```python
from build123d import *

# Parameters (mm, degrees)
CROQUIS1_W              = 66
CROQUIS1_H              = 62
SALIENTE_EXTRUIR1_DEPTH = 15
CROQUIS2_R              = 5
CROQUIS2_R_2            = 4
CORTAR_EXTRUIR1_DEPTH   = 15
CROQUIS3_R              = 7.5
CORTAR_EXTRUIR2_DEPTH   = 10


with BuildPart() as part:
    # Croquis1 → Saliente-Extruir1 (new body)
    with BuildSketch(Plane(origin=(0, 0, 0), x_dir=(1, 0, 0), z_dir=(0, 1, 0))):
        Rectangle(CROQUIS1_W, CROQUIS1_H)
    extrude(amount=SALIENTE_EXTRUIR1_DEPTH)

    # Croquis2 → Cortar-Extruir1 (cut)
    with BuildSketch(Plane(origin=(0, 15, 0), x_dir=(1, 0, 0), z_dir=(0, 1, 0))):
        with Locations((9, 0)):
            Circle(CROQUIS2_R)
        with Locations((-25, 0)):
            Circle(CROQUIS2_R_2)
        with Locations((25, 0)):
            Circle(CROQUIS2_R_2)
    extrude(amount=-CORTAR_EXTRUIR1_DEPTH, mode=Mode.SUBTRACT)

    # Croquis3 → Cortar-Extruir2 (cut)
    with BuildSketch(Plane(origin=(0, 15, 0), x_dir=(1, 0, 0), z_dir=(0, 1, 0))):
        with Locations((9, 0)):
            Circle(CROQUIS3_R)
    extrude(amount=-CORTAR_EXTRUIR2_DEPTH, mode=Mode.SUBTRACT)


solid = part.part
```
For this review, take the finished solid that the model builds, in its own axes (mm). A direction names the side the tool comes from. Coordinates: 2 decimals unless noted, no trailing zeros. Loops run counter-clockwise (first coordinate to the right, second up) from the corner with the lowest first, then second, coordinate; pieces in that order, holes last.
1. Add section A-A, the plane y = 8.25. Give the boundary of the cut face in (x, z), then the cut area to 3 significant figures.
2. Add section D-D, the plane x = 25. Give the boundary of the cut face in (y, z), then the cut area to 3 significant figures.
3. Add section C-C, the plane z = 0. Give the boundary of the cut face in (x, y).
4. Add section B-B, the plane x = 9. Give the boundary of the cut face in (y, z).
5. For faces 1 (the flat face through (14, 5, 2)), 2 (the flat face through (0, 15, 0)), list the 3-axis set-ups (+Z, -Z, +X, -X, +Y, -Y) from which the entire face can be reached by the end or side of a thin tool; tool diameter is ignored.
6. Insertion check: P1, Ø13, axis at x = 25, z = 0, coming from the -Y side; P2, Ø7.5, axis at x = 6.5, z = 2.5, coming from the +Y side. Each pin has a flat end and moves straight along its axis. Give the tip position at first contact, or say it passes through.
7. For line 1 (X direction, y = 11.75, z = 0); line 2 (X direction, y = 1.2, z = 0); line 3 (Z direction, x = -25, y = 6.75), list the stretches that pass through material, from the lowest coordinate up.
8. Mouldability with a two-part tool opening along Z and no side actions: class faces 3 (the flat face through (0, 7, 31)), 4 (the flat face through (-33, 7, 0)), 5 (the cylindrical face through (13.77, 2.54, -1.5)) as +Z half, -Z half, draft (parallel to the pull), parting line (faces both ways), or undercut.
Result:
1. outline: (-33, -31) - (33, -31) - (33, 31) - (-33, 31) - close; hole circle Ø8 at (-25, 0); hole circle Ø15 at (9, 0); hole circle Ø8 at (25, 0)
1. area: 3,810 mm2
2. outline: (0, -31) - (15, -31) - (15, -4) - (0, -4) - close; (0, 4) - (15, 4) - (15, 31) - (0, 31) - close
2. area: 810 mm2
3. outline: (-33, 0) - (-29, 0) - (-29, 15) - (-33, 15) - close; (-21, 0) - (4, 0) - (4, 5) - (1.5, 5) - (1.5, 15) - (-21, 15) - close; (14, 0) - (21, 0) - (21, 15) - (16.5, 15) - (16.5, 5) - (14, 5) - close; (29, 0) - (33, 0) - (33, 15) - (29, 15) - close
4. outline: (0, -31) - (15, -31) - (15, -7.5) - (5, -7.5) - (5, -5) - (0, -5) - close; (0, 5) - (5, 5) - (5, 7.5) - (15, 7.5) - (15, 31) - (0, 31) - close
5. face 1: +Y
5. face 2: +Z, -Z, +X, -X, +Y
6. P1: stops at y = 0
6. P2: stops at y = 5
7. line 1: x = -33 to -29, -21 to 1.5, 16.5 to 21, 29 to 33
7. line 2: x = -33 to -29, -21 to 4, 14 to 21, 29 to 33
7. line 3: z = -31 to -4, 4 to 31
8. face 3: +Z half
8. face 4: draft
8. face 5: undercut
